Part model, mm, in its own coordinate system. Give positions to 0.01 mm unless a question says otherwise; leave off trailing zeros. Loops run counter-clockwise (first coordinate to the right, second up) from the corner with the lowest first, then second, coordinate; pieces in that order, holes last. Notation, with made-up numbers: M -2,57 L 26,57 A29 cw 26,91 Z; hole C 55,33.25 d1. An arc over 180 degrees is marked long. Answer in a Markdown table with one row per item.
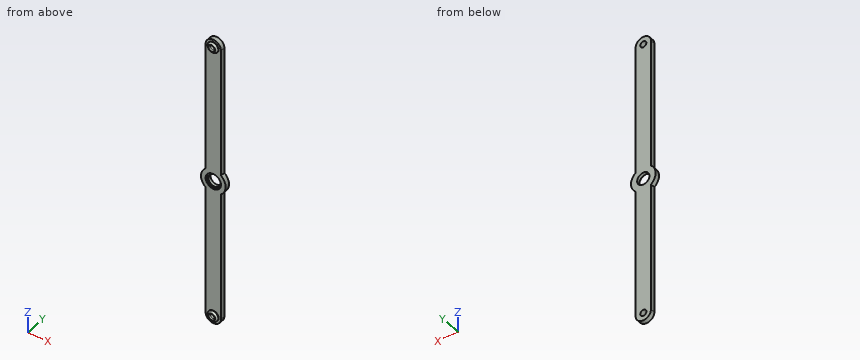
Autodesk Inventor part; units mm, degrees
ref_plane "YZ Plane" through (0, 0, 0) normal (1, 0, 0) x (0, 1, 0)
ref_plane "XZ Plane" through (0, 0, 0) normal (0, 1, 0) x (-1, 0, 0)
ref_plane "XY Plane" through (0, 0, 0) normal (0, 0, 1) x (1, 0, 0)
sketch "Эскиз1" plane through (0, 0, 0) normal (0, 1, 0) x (-1, 0, 0)
  circle A0 centre (0, 0) radius 2
  line L0 (0, 0) -> (0, -180) construction
  circle A1 centre (0, -180) radius 2
  arc A2 (5, 0) -> (-5, 0) centre (0, 0) ccw
  arc A3 (-5, -180) -> (5, -180) centre (0, -180) ccw
  line L1 (5, -180) -> (5, -96.245)
  line L2 (-5, -180) -> (-5, -96.245)
  line L3 (0, -90) -> (22.1641, -90) construction
  line L4 (5, -83.755) -> (5, 0)
  line L5 (-5, -83.755) -> (-5, 0)
  arc A4 (-5, -83.755) -> (-5, -96.245) centre (0, -90) ccw
  arc A5 (5, -96.245) -> (5, -83.755) centre (0, -90) ccw
  circle A6 centre (0, -90) radius 4
  dimension "d0" = 4
  dimension "d1" = 4
  dimension "d2" = 180
  dimension "d3" = 10
  dimension "d4" = 10
  dimension "d8" = 8
  dimension "d9" = 8
extrude "Выдавливание1" add sketch "Эскиз1" along normal blind 3
sketch "Эскиз2" plane through (0, 0, 0) normal (0, -1, 0) x (1, 0, 0)
  circle A0 centre (0, 0) radius 3.5
  circle A1 centre (0, -180) radius 2
  circle A2 centre (0, -180) radius 3.5
  circle A3 centre (0, 0) radius 2
  dimension "d10" = 7
  dimension "d11" = 7
extrude "Выдавливание2" add sketch "Эскиз2" along normal blind 1.5
chamfer "Фаска1" distance 1.2 angle 45 2 edges at (-3.5, -1.5, 0) (-3.5, -1.5, -180)
sketch "Эскиз3" plane through (0, 0, 0) normal (0, -1, 0) x (1, 0, 0)
  circle A0 centre (0, -90) radius 4
  circle A1 centre (0, -90) radius 5
  point P0 (0, 0)
  dimension "d17" = 10
extrude "Выдавливание3" cut sketch "Эскиз3" against normal blind 1
properties part number "04-02-Тяга"
(1) Drill centre lines: line 1 along Z through (x, y) = (0, 0.4); line 2 along Z through (x, y) = (-0.75, 1.4); line 3 along X through (y, z) = (1.95, -180). Where is each one in solid material? Low to high.
Recorded:
| item | result |
|---|---|
| line 1 | z = -185 to -182, -178 to -95, -85 to -2, 2 to 5 |
| line 2 | z = -184.94 to -181.85, -178.15 to -93.93, -86.07 to -1.85, 1.85 to 4.94 |
| line 3 | x = -5 to -2, 2 to 5 |
(2) Saw through at B-B (z = -90). Write the cut outline in (x, y), plus the area to 3 significant figures.
Recorded:
| item | result |
|---|---|
| outline | M -8,0 L -5,0 L -5,1 L -4,1 L -4,3 L -8,3 Z; M 4,1 L 5,1 L 5,0 L 8,0 L 8,3 L 4,3 Z |
| area | 22.0 mm^2 |
(3) Pin check, flat tips, straight feed: pin 1 Ø8 at (x, z) = (1.5, -157) entering from -Y; pin 2 Ø5 at (x, z) = (0.5, -91.5) entering from -Y; pin 3 Ø5 at (x, z) = (0, -180) entering from +Y; pin 4 Ø1.5 at (y, z) = (1.5, -157.5) entering from -X. Stop position of each tip, or through.
Recorded:
| item | result |
|---|---|
| pin 1 | stops at y = 0 |
| pin 2 | stops at y = 1 |
| pin 3 | stops at y = 3 |
| pin 4 | stops at x = -5 |
(4) Saw through at A-A (x = 0). Give the number of separate pieces and of enclosed holes in the cut face, plus the area to 3 significant figures.
Recorded:
| item | result |
|---|---|
| separate pieces | 4 |
| enclosed holes | 0 |
| area | 526 mm^2 |
